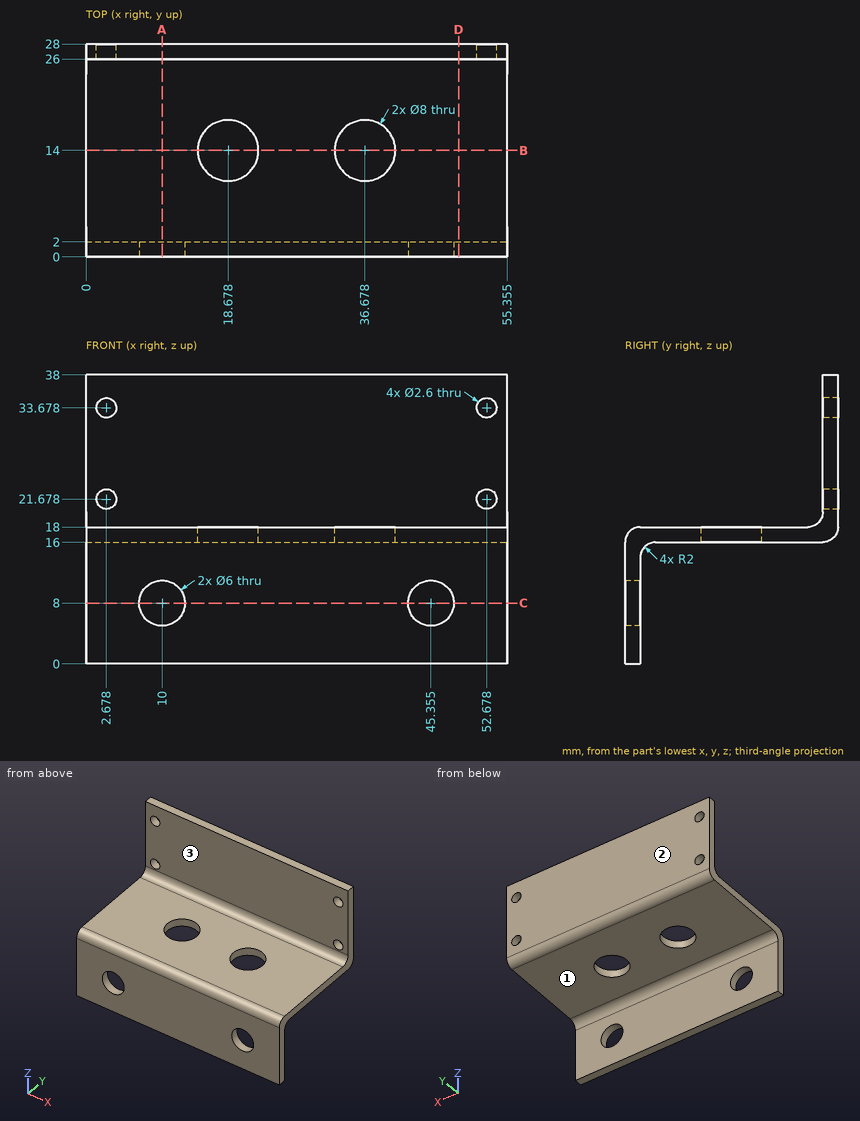
Geometry: see drawing. Coordinates: mm, zero at the bounding-box minimum. A direction names the side the tool comes from. Give positions to 0.01 mm unless a question says otherwise; leave off trailing zeros. Write each loop counter-clockwise with the first axis right and the second up, starting at its lowest first coordinate (ties: lowest second). Pieces come first, ordered by that corner, then holes. Notation, with made-up numbers: M 25,65 L 61,65 A22 cw 61,103 Z; hole C 24,17.25 d4. An arc over 180 degrees is marked long. Return JSON: item names as keys, results as strings. Group by question number.
1) Cut plane C-C, the plane z = 8. Output: boundary loops of the cut face in (x, y) (1 decimal).
2) Cut plane A-A, the plane x = 10. Output: boundary loops of the cut face in (y, z).
3) Cut plane D-D, the plane x = 49. Output: boundary loops of the cut face in (y, z), then the cut area to 3 significant figures.
4) Set-up query: the marked faces 1, 2 and 3. Return all of +Z, -Z, +X, -X, +Y, -Y with unobstructed straight access to the full face (end or side cutting, diameter ignored); none if empty.
5) First-contact query: pin 1 Ø3 at (x, z) = (52.68, 21.68) entering from -Y; pin 2 Ø10.5 at (x, y) = (36.68, 14) entering from -Z; pin 3 Ø4 at (x, z) = (41, 4) entering from +Y. Flat tips, straight axial feed; report the tip coordinate or a pass-through.
6) Ray query, L1, parallel to Z at x = 10, y = 8.75; L2, parallel to Y at x = 19, z = 10.5; L3, parallel to Y at x = 24, z = 21. Return the intervals inside material, ascending.
7) Cut plane B-B, the plane y = 14. Output: boundary loops of the cut face in (x, z) (1 decimal).
Data:
{
 "1": {"outline": "M 0,0 L 7,0 L 7,2 L 0,2 Z; M 13,0 L 42.4,0 L 42.4,2 L 13,2 Z; M 48.4,0 L 55.4,0 L 55.4,2 L 48.4,2 Z"},
 "2": {"outline": "M 0,0 L 2,0 L 2,5 L 0,5 Z; M 0,11 L 2,11 L 2,14 A2 cw 4,16 L 26,16 A2 ccw 28,18 L 28,38 L 26,38 L 26,20 A2 cw 24,18 L 2,18 A2 ccw 0,16 Z"},
 "3": {"outline": "M 0,0 L 2,0 L 2,14 A2 cw 4,16 L 26,16 A2 ccw 28,18 L 28,38 L 26,38 L 26,20 A2 cw 24,18 L 2,18 A2 ccw 0,16 Z", "area": "128 mm²"},
 "4": {"face 1": "-Z, +X, -X, +Y", "face 2": "+Z, -Z, +X, -X, +Y", "face 3": "+Z, +X, -X, -Y"},
 "5": {"pin 1": "stops at y = 26", "pin 2": "stops at z = 16", "pin 3": "stops at y = 2"},
 "6": {"L1": "z = 16 to 18", "L2": "y = 0 to 2", "L3": "y = 26 to 28"},
 "7": {"outline": "M 0,16 L 14.7,16 L 14.7,18 L 0,18 Z; M 22.7,16 L 32.7,16 L 32.7,18 L 22.7,18 Z; M 40.7,16 L 55.4,16 L 55.4,18 L 40.7,18 Z"}
}
